Can you work these out from the model? Positions are in its coordinate system, mm. Face numbers are marked on the shaded views. A direction names the side the tool comes from. Coordinates: 2 decimals unless noted, no trailing zeros. Order: outer loops, then holes, each group sorted by start corner. A loop starts at its lowest first (then second) coordinate and runs counter-clockwise, first axis right, second up. Notation, with made-up numbers: (-28, 78.5) -> (-12, 78.5) arc R10 cw to (-12, 82.5) -> close; hole circle Ø6 at (-6, 75.25). An arc over 180 degrees is marked (long way). Answer in a Markdown table with one row per item. Add a question column.
1. Will this pin go through, and if not, where does the flat tip stop? pin 1 (5 mm diameter, centred on y = 7.5, z = -6.5, fed in from +X).
2. Imagine slicing it at D-D on y = 1. Write out the boundary of the cut face in (x, z).
3. Imagine slicing it at C-C on x = -10. Write out the boundary of the cut face in (y, z).
4. Imagine slicing it at B-B on z = 6.5. Write out the boundary of the cut face in (x, y).
5. If I drill on line 1 along Z through (x, y) = (-4.75, 11.25); line 2 along X through (y, z) = (8, 1); line 3 along X through (y, z) = (3.75, -3), over which ranges is the centre line in solid material (lowest first)? Write a range as [from, to].
6. On a 3-axis mill with a long thin cutter (end or side, diameter ignored), from which of +Z, -Z, +X, -X, +Y, -Y can I reach the whole of each face in a straight line? I mean the marked faces 4, 5 and 6. Say none if no direction works.
7. Imagine slicing it at A-A on x = 7.4. Write out the boundary of the cut face in (y, z), plus the area to 3 significant figures.
8. We'd pull the mould along Y, two halves only. Please class the marked faces 1, 2 and 3: pulls with the +Y half, pulls with the -Y half, needs draft (parallel to the pull), parting line crosses it, or undercut.
from build123d import *

# Parameters (mm, degrees)
SKETCH1_W             = 25
SKETCH1_H             = 25
BOSS_EXTRUDE1_DEPTH   = 15
SKETCH2_W             = 11.4
SKETCH2_H             = 19
CUT_EXTRUDE1_DEPTH    = 16
M3_CLEARANCE_HOLE1_D  = 3
FOR_M4_HEAT_SET_D     = 5.6134
FOR_M4_HEAT_SET_DEPTH = 8.1
FILLET1_R             = 0.5


with BuildPart() as part:
    # Sketch1 → Boss-Extrude1 (new body)
    with BuildSketch(Plane(origin=(0, 0, 0), x_dir=(1, 0, 0), z_dir=(0, 1, 0))):
        Rectangle(SKETCH1_W, SKETCH1_H)
    extrude(amount=BOSS_EXTRUDE1_DEPTH)

    # Sketch2 → Cut-Extrude1 (cut, through all)
    with BuildSketch(Plane(origin=(0, 15, 0), x_dir=(1, 0, 0), z_dir=(0, 1, 0))):
        with Locations((-1.3, 0)):
            Rectangle(SKETCH2_W, SKETCH2_H)
    extrude(amount=-CUT_EXTRUDE1_DEPTH, mode=Mode.SUBTRACT)

    # M3 Clearance Hole1 (through all)
    with Locations(Plane(origin=(0, 15, 0), x_dir=(1, 0, 0), z_dir=(0, 1, 0))):
        with Locations((-10, 0), (7.4, 0)):
            Hole(M3_CLEARANCE_HOLE1_D / 2)

    # for m4 heat set
    with Locations(Plane(origin=(12.5, 0, 0), x_dir=(0, 0, -1), z_dir=(1, 0, 0))):
        with Locations((-6.5, 7.5), (6.5, 7.5)):
            Hole(FOR_M4_HEAT_SET_D / 2, depth=FOR_M4_HEAT_SET_DEPTH)

    # Fillet1
    fillet1_edges = [part.edges().sort_by_distance(p)[0] for p in [
        (-7, 7.5, 9.5),
        (-7, 7.5, -9.5),
        (4.4, 7.5, -9.5),
        (4.4, 7.5, 9.5),
    ]]
    fillet(fillet1_edges, radius=FILLET1_R)


solid = part.part
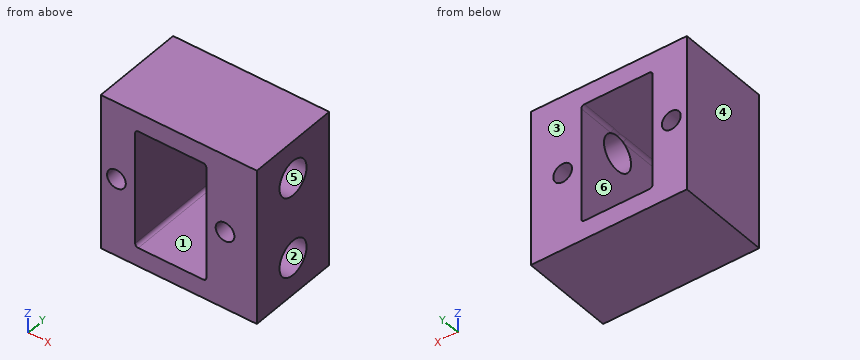
Answers follow:
| question | item | result |
|---|---|---|
| 1 | pin 1 | stops at x = -7 |
| 2 | outline | (-12.5, -12.5) -> (12.5, -12.5) -> (12.5, 12.5) -> (-12.5, 12.5) -> close; hole circle Ø3 at (-10, 0); hole (-7, -9) arc R0.5 ccw to (-6.5, -9.5) -> (3.9, -9.5) arc R0.5 ccw to (4.4, -9) -> (4.4, 9) arc R0.5 ccw to (3.9, 9.5) -> (-6.5, 9.5) arc R0.5 ccw to (-7, 9) -> close; hole circle Ø3 at (7.4, 0) |
| 3 | outline | (0, -12.5) -> (15, -12.5) -> (15, -1.5) -> (0, -1.5) -> close; (0, 1.5) -> (15, 1.5) -> (15, 12.5) -> (0, 12.5) -> close |
| 4 | outline | (-12.5, 0) -> (-7, 0) -> (-7, 15) -> (-12.5, 15) -> close; (4.4, 0) -> (12.5, 0) -> (12.5, 4.69) -> (4.4, 4.69) -> close; (4.4, 10.31) -> (12.5, 10.31) -> (12.5, 15) -> (4.4, 15) -> close |
| 5 | line 1 | z = [-12.5, -9.5], [9.5, 12.5] |
| 5 | line 2 | x = [-12.5, -11.12], [-8.88, -7], [4.4, 6.28], [8.52, 12.5] |
| 5 | line 3 | x = [-12.5, -7], [4.4, 12.5] |
| 6 | face 4 | +Z, -Z, -X, +Y, -Y |
| 6 | face 5 | +X |
| 6 | face 6 | +Y, -Y |
| 7 | outline | (0, -12.5) -> (15, -12.5) -> (15, -1.5) -> (0, -1.5) -> close; (0, 1.5) -> (15, 1.5) -> (15, 12.5) -> (0, 12.5) -> close; hole circle Ø5.61 at (7.5, -6.5); hole circle Ø5.61 at (7.5, 6.5) |
| 7 | area | 281 mm² |
| 8 | face 1 | needs draft |
| 8 | face 2 | undercut |
| 8 | face 3 | pulls with the +Y half |
